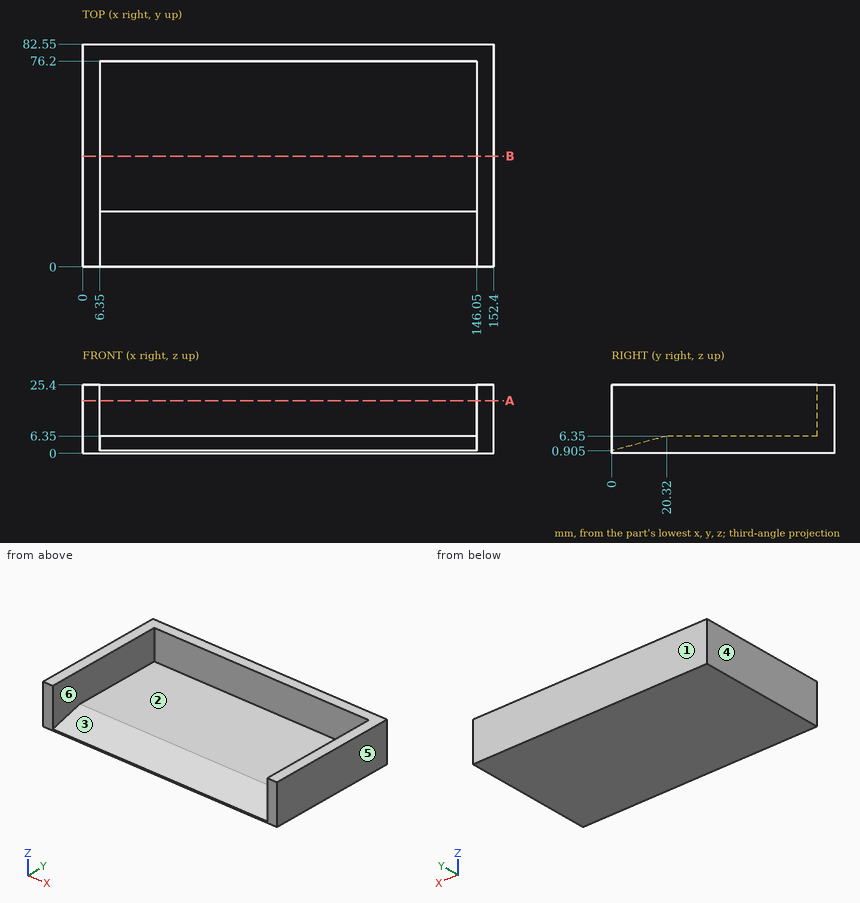
Geometry: see drawing. Coordinates: mm, zero at the bounding-box minimum. A direction names the side the tool comes from. Coordinates: 2 decimals unless noted, no trailing zeros. Loops run counter-clockwise (first coordinate to the right, second up) from the corner with the lowest first, then second, coordinate; pieces in that order, holes last.
Q1. Cut plane B-B (y = 41). Output: boundary loops of the cut face in (x, z), then the cut area to 3 significant figures.
Q2. Draft query along X for the marked faces 3, 4, 5 and 6. Return one class per face: +X half, -X half, draft (parallel to the pull), parting line (faces both ways), or undercut.
Q3. Set-up query: the marked faces 1 and 2. Return all of +Z, -Z, +X, -X, +Y, -Y with unobstructed straight access to the full face (end or side cutting, diameter ignored); none if empty.
Q4. Cut plane A-A (z = 19.5). Output: boundary loops of the cut face in (x, y), then the cut area to 3 significant figures.
Q5. Contact query for a flat-ended pin moving along its axis: pin 1 (3 mm diameter, centred on x = 19.5, z = 17, fed in from -Y). Output: stop coordinate, or through.
Q6. Material intervals for line 1 (X direction, y = 37.5, z = 21.25); line 2 (Z direction, x = 88.5, y = 62.5); line 3 (Y direction, x = 84, z = 10.75), sorted ascending.
Working result:
1. outline: (0, 0) - (152.4, 0) - (152.4, 25.4) - (146.05, 25.4) - (146.05, 6.35) - (6.35, 6.35) - (6.35, 25.4) - (0, 25.4) - close
1. area: 1,210 mm2
2. face 3: undercut
2. face 4: -X half
2. face 5: +X half
2. face 6: undercut
3. face 1: +Z, -Z, +X, -X, +Y
3. face 2: +Z, -Y
4. outline: (0, 0) - (6.35, 0) - (6.35, 76.2) - (146.05, 76.2) - (146.05, 0) - (152.4, 0) - (152.4, 82.55) - (0, 82.55) - close
4. area: 1,940 mm2
5. pin 1: stops at y = 76.2
6. line 1: x = 0 to 6.35, 146.05 to 152.4
6. line 2: z = 0 to 6.35
6. line 3: y = 76.2 to 82.55
